Source: CAD feature listing. Evaluate the final solid. Frame: model axes, mm. Face numbers are marked on the shaded views. A direction names the side the tool comes from. Give positions to 0.01 mm unless a question says otherwise; leave off trailing zeros. Loops run counter-clockwise (first coordinate to the right, second up) from the corner with the lowest first, then second, coordinate; pieces in that order, holes last.
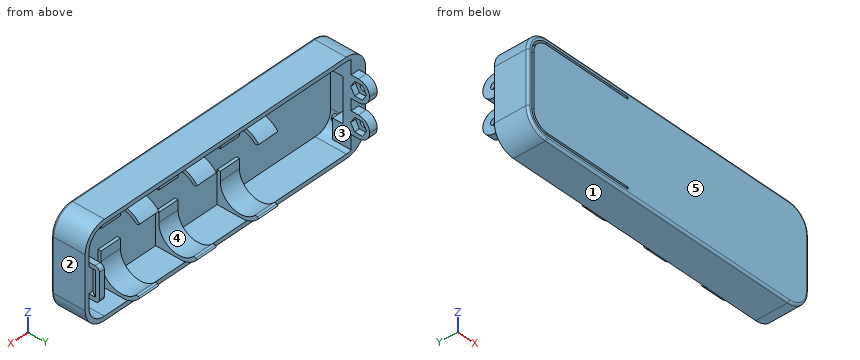
from build123d import *

# Parameters (mm, degrees)
BOSS_EXTRUDE1_DEPTH    = 2
BOSS_EXTRUDE2_DEPTH    = 14
FILLET1_R              = 1
SKETCH3_W              = 10
SKETCH3_H              = 41
BOSS_EXTRUDE3_DEPTH    = 25
BOSS_EXTRUDE5_DEPTH    = 12.75
CUT_EXTRUDE3_DEPTH     = 2.5
CUT_EXTRUDE5_OUTLINE_R = 1.5
CUT_EXTRUDE5_DEPTH     = 5.5
SKETCH10_W             = 2.5
SKETCH10_H             = 16
BOSS_EXTRUDE6_DEPTH    = 19
CUT_EXTRUDE6_DEPTH     = 12
FILLET2_R              = 2
CUT_EXTRUDE7_START     = -8.75
CUT_EXTRUDE7_DEPTH     = 8.75
CUT_EXTRUDE13_DEPTH    = 84
CUT_EXTRUDE15_DEPTH    = 2
BOSS_EXTRUDE7_START    = 4.9
BOSS_EXTRUDE7_DEPTH    = 4.9
SKETCH17_R             = 1.4
BOSS_EXTRUDE8_DEPTH    = 2
FILLET3_R              = 0.25
CUT_EXTRUDE16_START    = -42
CUT_EXTRUDE16_DEPTH    = 42
FILLET4_R              = 1


# Read off the part's stored shape, not the designer's step: Cut-Extrude5
with BuildPart() as part:
    # Sketch1 → Boss-Extrude1 (new body)
    with BuildSketch(Plane(origin=(0, 0, 0), x_dir=(1, 0, 0), z_dir=(0, 1, 0))):
        with BuildLine():
            Line((-10, 0), (-136, 0))
            ThreePointArc((-136, 0), (-143.071067812, -2.928932188), (-146, -10))
            Line((-146, -10), (-146, -35))
            ThreePointArc((-146, -35), (-143.071067812, -42.071067812), (-136, -45))
            Line((-136, -45), (-10, -45))
            ThreePointArc((-10, -45), (-2.928932188, -42.071067812), (0, -35))
            Line((0, -35), (0, -10))
            ThreePointArc((0, -10), (-2.928932188, -2.928932188), (-10, 0))
        make_face()
    extrude(amount=BOSS_EXTRUDE1_DEPTH)

    # Sketch2 → Boss-Extrude2 (add)
    with BuildSketch(Plane(origin=(0, 2, 0), x_dir=(1, 0, 0), z_dir=(0, 1, 0))):
        with BuildLine():
            Line((-10, 0), (-136, 0))
            ThreePointArc((-136, 0), (-143.071067812, -2.928932188), (-146, -10))
            Line((-146, -10), (-146, -35))
            ThreePointArc((-146, -35), (-143.071067812, -42.071067812), (-136, -45))
            Line((-136, -45), (-10, -45))
            ThreePointArc((-10, -45), (-2.928932188, -42.071067812), (0, -35))
            Line((0, -35), (0, -10))
            ThreePointArc((0, -10), (-2.928932188, -2.928932188), (-10, 0))
        make_face()
        with BuildLine():
            Line((-10, -2), (-136, -2))
            ThreePointArc((-136, -2), (-141.656854249, -4.343145751), (-144, -10))
            Line((-144, -10), (-144, -35))
            ThreePointArc((-144, -35), (-141.656854249, -40.656854249), (-136, -43))
            Line((-136, -43), (-10, -43))
            ThreePointArc((-10, -43), (-4.343145751, -40.656854249), (-2, -35))
            Line((-2, -35), (-2, -10))
            ThreePointArc((-2, -10), (-4.343145751, -4.343145751), (-10, -2))
        make_face(mode=Mode.SUBTRACT)
    extrude(amount=BOSS_EXTRUDE2_DEPTH)

    # Fillet1
    fillet1_edges = [part.edges().sort_by_distance(p)[0] for p in [
        (-73, 0, 0),
        (-2.928932188, 0, 2.928932188),
        (0, 0, 22.5),
        (-2.928932188, 0, 42.071067812),
        (-73, 0, 45),
        (-143.071067812, 0, 42.071067812),
        (-146, 0, 22.5),
        (-143.071067812, 0, 2.928932188),
    ]]
    fillet(fillet1_edges, radius=FILLET1_R)

    # Sketch3 → Boss-Extrude3 (add)
    with BuildSketch(Plane(origin=(0, 2, 0), x_dir=(1, 0, 0), z_dir=(0, 1, 0))):
        with Locations((-57, -22.5)):
            Rectangle(SKETCH3_W, SKETCH3_H)
        with Locations((-89, -22.5)):
            Rectangle(SKETCH3_W, SKETCH3_H)
        with Locations((-27, -22.5)):
            Rectangle(SKETCH3_W, SKETCH3_H)
    extrude(amount=BOSS_EXTRUDE3_DEPTH)

    # Sketch7 → Boss-Extrude5 (add)
    with BuildSketch(Plane(origin=(0, 12, 0), x_dir=(1, 0, 0), z_dir=(0, 1, 0))):
        with BuildLine():
            ThreePointArc((-138.5, -2.400657923), (-142.480740698, -5.30958424), (-144, -10))
            Line((-144, -10), (-144, -35))
            ThreePointArc((-144, -35), (-142.480740698, -39.69041576), (-138.5, -42.599342077))
            Line((-138.5, -42.599342077), (-138.5, -2.400657923))
        make_face()
    extrude(amount=BOSS_EXTRUDE5_DEPTH)

    # Sketch8 → Cut-Extrude3 (cut)
    with BuildSketch(Plane(origin=(-138.5, 0, 0), x_dir=(0, 0, -1), z_dir=(1, 0, 0))):
        Polygon((-27.25, 17.620834875), (-27.25, 21.373611625), (-30.5, 23.25), (-33.75, 21.373611625), (-33.75, 17.620834875), (-30.5, 15.744446501), align=None)
        Polygon((-11.25, 17.620834875), (-11.25, 21.373611625), (-14.5, 23.25), (-17.75, 21.373611625), (-17.75, 17.620834875), (-14.5, 15.744446501), align=None)
    extrude(amount=-CUT_EXTRUDE3_DEPTH, mode=Mode.SUBTRACT)

    # Cut-Extrude5 outline → Cut-Extrude5 (cut)
    with BuildSketch(Plane(origin=(-144, 0, 0), x_dir=(0, 0, -1), z_dir=(1, 0, 0))):
        with BuildLine():
            Line((-2.400657923, 24.75), (-14.500000003, 24.75))
            ThreePointArc((-14.500000003, 24.75), (-10.785725941, 23.211497311), (-9.24722325, 19.49722325))
            Line((-9.24722325, 19.49722325), (-9.24722325, 16))
            Line((-9.24722325, 16), (-2.400657923, 16))
            Line((-2.400657923, 16), (-2.400657923, 24.75))
        make_face()
        with BuildLine():
            ThreePointArc((-19.75277675, 19.49722325), (-18.214274061, 23.211497309), (-14.500000003, 24.75))
            Line((-14.500000003, 24.75), (-30.49999999, 24.75))
            ThreePointArc((-30.49999999, 24.75), (-26.785725937, 23.211497307), (-25.24722325, 19.49722325))
            Line((-25.24722325, 19.49722325), (-25.24722325, 16))
            Line((-25.24722325, 16), (-19.75277675, 16))
            Line((-19.75277675, 16), (-19.75277675, 19.49722325))
        make_face()
        with BuildLine():
            ThreePointArc((-35.75277675, 19.49722325), (-34.214274056, 23.211497313), (-30.49999999, 24.75))
            Line((-30.49999999, 24.75), (-42.599342077, 24.75))
            Line((-42.599342077, 24.75), (-42.599342077, 16))
            Line((-42.599342077, 16), (-35.75277675, 16))
            Line((-35.75277675, 16), (-35.75277675, 19.49722325))
        make_face()
        with Locations((-14.5, 19.49722325)):
            Circle(CUT_EXTRUDE5_OUTLINE_R)
        with Locations((-30.5, 19.49722325)):
            Circle(CUT_EXTRUDE5_OUTLINE_R)
    extrude(amount=CUT_EXTRUDE5_DEPTH, mode=Mode.SUBTRACT)

    # Sketch10 → Boss-Extrude6 (add)
    with BuildSketch(Plane(origin=(0, 2, 0), x_dir=(1, 0, 0), z_dir=(0, 1, 0))):
        with Locations((-3.25, -22.5)):
            Rectangle(SKETCH10_W, SKETCH10_H)
    extrude(amount=BOSS_EXTRUDE6_DEPTH)

    # Sketch11 → Cut-Extrude6 (cut)
    with BuildSketch(Plane(origin=(0, 0, 16.5), x_dir=(-1, 0, 0), z_dir=(0, 0, -1))):
        Polygon((2, 19), (4, 16), (2, 16), align=None)
    extrude(amount=-CUT_EXTRUDE6_DEPTH, mode=Mode.SUBTRACT)

    # Fillet2
    fillet2_edges = [part.edges().sort_by_distance(p)[0] for p in [
        (-3.25, 21, 14.5),
        (-3.25, 21, 30.5),
    ]]
    fillet(fillet2_edges, radius=FILLET2_R)

    # Sketch12 → Cut-Extrude7 (cut)
    with BuildSketch(Plane(origin=(0, 24.75, 0), x_dir=(1, 0, 0), z_dir=(0, 1, 0)).offset(CUT_EXTRUDE7_START)):
        with BuildLine():
            ThreePointArc((-143.964504201, -9.24722325), (-143.991121123, -9.623193423), (-144, -10))
            Line((-144, -10), (-144, -19.75277675))
            Line((-144, -19.75277675), (-142.5, -19.75277675))
            Line((-142.5, -19.75277675), (-142.5, -9.24722325))
            Line((-142.5, -9.24722325), (-143.964504201, -9.24722325))
        make_face()
        with BuildLine():
            ThreePointArc((-144, -35), (-143.991121123, -35.376806577), (-143.964504201, -35.75277675))
            Line((-143.964504201, -35.75277675), (-142.5, -35.75277675))
            Line((-142.5, -35.75277675), (-142.5, -25.24722325))
            Line((-142.5, -25.24722325), (-144, -25.24722325))
            Line((-144, -25.24722325), (-144, -35))
        make_face()
    extrude(amount=CUT_EXTRUDE7_DEPTH, mode=Mode.SUBTRACT)

    # Sketch4 → Cut-Extrude13 (cut)
    with BuildSketch(Plane.ZY.offset(22)):
        with BuildLine():
            Line((6, 21.806957477), (7.088888889, 20.436986314))
            ThreePointArc((7.088888889, 20.436986314), (4.030569417, 9.86961424), (13, 3.5))
            Line((13, 3.5), (17.5, 3.5))
            Line((17.5, 3.5), (17.5, 2))
            Line((17.5, 2), (27.5, 2))
            Line((27.5, 2), (27.5, 3.5))
            Line((27.5, 3.5), (32, 3.5))
            ThreePointArc((32, 3.5), (40.969430583, 9.86961424), (37.911111111, 20.436986314))
            Line((37.911111111, 20.436986314), (39, 21.806957477))
            ThreePointArc((39, 21.806957477), (41.560108062, 18.930163053), (43, 15.358495283))
            Line((43, 15.358495283), (43, 27))
            Line((43, 27), (2, 27))
            Line((2, 27), (2, 15.358495283))
            ThreePointArc((2, 15.358495283), (3.439891938, 18.930163053), (6, 21.806957477))
        make_face()
    extrude(amount=CUT_EXTRUDE13_DEPTH, mode=Mode.SUBTRACT)

    # Sketch15 → Cut-Extrude15 (cut)
    with BuildSketch(Plane.XZ):
        with BuildLine():
            Line((-136, 2), (-94, 2))
            Line((-94, 2), (-94, 3))
            Line((-94, 3), (-95, 3))
            Line((-95, 3), (-136, 3))
            ThreePointArc((-136, 3), (-140.949747468, 5.050252532), (-143, 10))
            Line((-143, 10), (-143, 35))
            ThreePointArc((-143, 35), (-140.949747468, 39.949747468), (-136, 42))
            Line((-136, 42), (-95, 42))
            Line((-95, 42), (-94, 42))
            Line((-94, 42), (-94, 43))
            Line((-94, 43), (-136, 43))
            ThreePointArc((-136, 43), (-141.656854249, 40.656854249), (-144, 35))
            Line((-144, 35), (-144, 10))
            ThreePointArc((-144, 10), (-141.656854249, 4.343145751), (-136, 2))
        make_face()
    extrude(amount=-CUT_EXTRUDE15_DEPTH, mode=Mode.SUBTRACT)

    # Sketch16 → Boss-Extrude7 (add)
    with BuildSketch(Plane.XZ.offset(-12).offset(BOSS_EXTRUDE7_START)):
        with BuildLine():
            Line((-144, 35), (-144, 33))
            Line((-144, 33), (-138.5, 33))
            Line((-138.5, 33), (-138.5, 42.599342077))
            ThreePointArc((-138.5, 42.599342077), (-142.480740698, 39.69041576), (-144, 35))
        make_face()
        with BuildLine():
            Line((-138.5, 12), (-144, 12))
            Line((-144, 12), (-144, 10))
            ThreePointArc((-144, 10), (-142.480740698, 5.30958424), (-138.5, 2.400657923))
            Line((-138.5, 2.400657923), (-138.5, 12))
        make_face()
    extrude(amount=-BOSS_EXTRUDE7_DEPTH)

    # Sketch17 → Boss-Extrude8 (add)
    with BuildSketch(Plane.XZ.offset(-7.1)):
        with Locations(Location((-141.25, 35.2, 0), (0, 0, 270))):
            Circle(SKETCH17_R)
        with Locations(Location((-141.25, 9.8, 0), (0, 0, 270))):
            Circle(SKETCH17_R)
    extrude(amount=BOSS_EXTRUDE8_DEPTH)

    # Fillet3
    fillet3_edges = [part.edges().sort_by_distance(p)[0] for p in [
        (-141.25, 5.1, 36.6),
        (-141.25, 5.1, 11.2),
    ]]
    fillet(fillet3_edges, radius=FILLET3_R)

    # Sketch19 → Cut-Extrude16 (cut)
    with BuildSketch(Plane.ZY.offset(94).offset(CUT_EXTRUDE16_START)):
        with BuildLine():
            Line((42, 5.72527161), (40.024254166, 7.914594894))
            ThreePointArc((40.024254166, 7.914594894), (39.435774802, 7.087364962), (38.762381995, 6.327654854))
            Line((38.762381995, 6.327654854), (40, 4.956250765))
            Line((40, 4.956250765), (40, 2.5))
            Line((40, 2.5), (42, 2.5))
            Line((42, 2.5), (42, 5.72527161))
        make_face()
    extrude(amount=CUT_EXTRUDE16_DEPTH, mode=Mode.SUBTRACT)

    # Fillet4
    fillet4_edges = [part.edges().sort_by_distance(p)[0] for p in [
        (-57, 20.436986314, 7.088888889),
        (-89, 20.436986314, 7.088888889),
        (-27, 20.436986314, 7.088888889),
        (-57, 20.436986314, 37.911111111),
        (-89, 20.436986314, 37.911111111),
        (-27, 20.436986314, 37.911111111),
    ]]
    fillet(fillet4_edges, radius=FILLET4_R)


solid = part.part
1) Pull-direction query (Z, two-part tool) for the marked faces 1, 2 and 3; classes: released by +Z, released by -Z, zero draft, split by the parting line, or undercut.
Checks:
face 1: released by -Z
face 2: zero draft
face 3: undercut
2) Cut plane A-A (x = -134). Return loops of the section in (y, z).
Checks:
outline: (0, 1) arc R1 ccw to (1, 0) - (16, 0) - (16, 2) - (0, 2) - close; (0, 3) - (2, 3) - (2, 42) - (0, 42) - close; (0, 43) - (16, 43) - (16, 45) - (1, 45) arc R1 ccw to (0, 44) - close
3) Contact query for flat-ended pins moving along their axis: P1, Ø2, axis at x = -28, z = 31, coming from the +Y side; P2, Ø2, axis at x = -140.5, y = 20.5, coming from the -Z side; P3, Ø4, axis at x = -142.5, y = 9, coming from the +Z side; P4, Ø3, axis at x = -41.5, y = 19, coming from the +Z side. Output: stop coordinate, or through.
Checks:
P1: stops at y = 3.5
P2: stops at z = 9.25
P3: stops at z = 43.93
P4: passes through
4) Cut plane C-C (x = -91). Return loops of the section in (y, z), and give its area (3 significant figures).
Checks:
outline: (0, 1) arc R1 ccw to (1, 0) - (16, 0) - (16, 2) - (15.36, 2) arc R11.25 ccw to (21.81, 6) - (21.18, 6.5) arc R1 ccw to (19.84, 6.41) arc R9.5 cw to (3.5, 13) - (3.5, 17.5) - (2, 17.5) - (2, 27.5) - (3.5, 27.5) - (3.5, 32) arc R9.5 cw to (6.33, 38.76) - (4.96, 40) - (2.5, 40) - (2.5, 42) - (5.73, 42) - (7.91, 40.02) arc R9.5 cw to (19.84, 38.59) arc R1 ccw to (21.18, 38.5) - (21.81, 39) arc R11.25 ccw to (15.36, 43) - (16, 43) - (16, 45) - (1, 45) arc R1 ccw to (0, 44) - close
area: 280 mm2
5) Ray query, probe 1 along Y at (x, z) = (-141.5, 30.5); probe 2 along X at (y, z) = (7.25, 18.5); probe 3 along X at (y, z) = (12.25, 14). Return the intervals inside material, ascending.
Checks:
probe 1: y = 0 to 2, 12 to 18, 21 to 24.75
probe 2: x = -146 to -144, -4.5 to 0
probe 3: x = -146 to -138.5, -2 to 0
6) Reachability of the marked faces 4 and 5 from +Z, -Z, +X, -X, +Y, -Y: full face, straight path, thin tool, end or side. Return the list, or none.
Checks:
face 4: none
face 5: +Z, -Z, +X, -X, -Y
7) Cut plane B-B (x = -38.5). Return loops of the section in (y, z).
Checks:
outline: (0, 1) arc R1 ccw to (1, 0) - (16, 0) - (16, 2) - (2, 2) - (2, 43) - (16, 43) - (16, 45) - (1, 45) arc R1 ccw to (0, 44) - close
